Input: part model. Units: mm. Frame: model coordinates. Coordinates: 2 decimals unless noted, no trailing zeros. Write each loop counter-clockwise with the first axis right and the second up, starting at its lowest first coordinate (ties: lowest second). Pieces come first, ordered by that corner, then holes. Notation, with made-up numbers: (-12, 29.5) - (1, 29.5) arc R26 ccw to (1, 66.5) - close; hole circle Ø3 at (37.5, -26.75). An arc over 180 degrees is marked (long way). Put each result on its own line as item: value. Start each with the question number.
1. Line query: line 1 (Y direction, x = 2.75, z = -0.25); line 2 (X direction, y = 2, z = -8) (3 decimals); line 3 (Z direction, x = 1, y = 28.5). Output: solid intervals per line, ascending.
2. Pin query (flat end, axial travel): pin 1 (1.5 mm diameter, centred on x = 2, z = -4, fed in from -Y) (3 decimals). Return the tip coordinate at first contact, or that it passes through.
3. Cut plane A-A, the plane x = 1.3. Return loops of the section in (y, z).
4. Cut plane B-B, the plane y = 29. Return loops of the section in (x, z) (1 decimal), and give its area (3 significant figures).
5. Cut plane C-C, the plane z = -2.25. Return loops of the section in (x, y) (3 decimals).
6. Cut plane D-D, the plane y = 17. Return loops of the section in (x, z) (3 decimals), and give its area (3 significant figures).
from build123d import *

# Parameters (mm, degrees)
BOSS_EXTRUDE1_DEPTH = 31.75
SKETCH7_W           = 3.6195
SKETCH7_H           = 6.35
CUT_EXTRUDE2_DEPTH  = 3.8575
SKETCH10_W          = 3.6195
SKETCH10_H          = 6.35
CUT_EXTRUDE4_DEPTH  = 3.8575
SKETCH15_R          = 1.6383
CUT_EXTRUDE5_DEPTH  = 3.8575


with BuildPart() as part:
    # Sketch3 → Boss-Extrude1 (new body)
    with BuildSketch(Plane(origin=(0, 0, 0), x_dir=(1, 0, 0), z_dir=(0, 1, 0))):
        with BuildLine():
            Line((0.635, 9.525), (0, 9.525))
            Line((0, 9.525), (0, 0))
            ThreePointArc((0, 0), (2.652258403, -0.737803327), (0.762, 1.263634045))
            Line((0.762, 1.263634045), (0.762, 0.430677954))
            ThreePointArc((0.762, 0.430677954), (2.190088254, -0.224506403), (0.635, 0))
            Line((0.635, 0), (0.635, 9.525))
        make_face()
    extrude(amount=BOSS_EXTRUDE1_DEPTH)

    # Sketch7 → Cut-Extrude2 (cut, through all)
    with BuildSketch(Plane(origin=(0, 0, 0), x_dir=(0, 0, -1), z_dir=(1, 0, 0))):
        with Locations((0, 34.925)):
            Rectangle(SKETCH7_W, SKETCH7_H)
        with Locations((0, 9.525)):
            Rectangle(SKETCH7_W, SKETCH7_H)
        with Locations((0, 22.225)):
            Rectangle(SKETCH7_W, SKETCH7_H)
    extrude(amount=CUT_EXTRUDE2_DEPTH, mode=Mode.SUBTRACT)

    # Sketch10 → Cut-Extrude4 (cut, through all)
    with BuildSketch(Plane(origin=(0, 0, 0), x_dir=(0, 0, -1), z_dir=(1, 0, 0))):
        with Locations((0, 15.875)):
            Rectangle(SKETCH10_W, SKETCH10_H)
    extrude(amount=CUT_EXTRUDE4_DEPTH, mode=Mode.SUBTRACT)

    # Sketch15 → Cut-Extrude5 (cut, through all)
    with BuildSketch(Plane(origin=(0, 0, 0), x_dir=(0, 0, -1), z_dir=(1, 0, 0))):
        with Locations((5.9436, 3.175)):
            Circle(SKETCH15_R)
    cut_extrude5 = extrude(amount=CUT_EXTRUDE5_DEPTH, mode=Mode.SUBTRACT)

    # Mirror1: Cut-Extrude5 across plane
    add(cut_extrude5.mirror(Plane(origin=(0, 15.875, 0), x_dir=(0, 0, 1), z_dir=(0, -1, 0))), mode=Mode.SUBTRACT)


solid = part.part
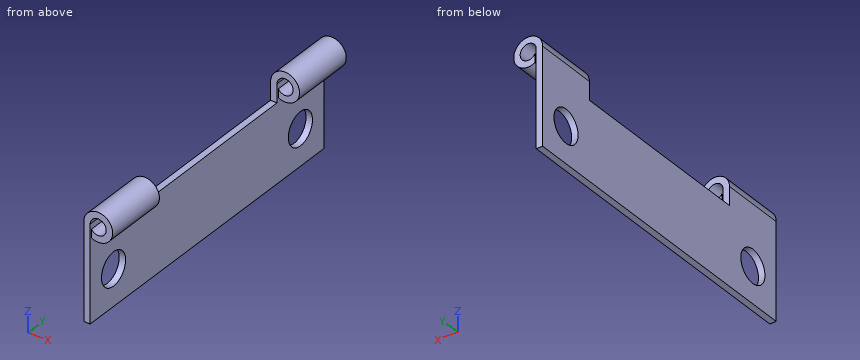
Report:
1. line 1: y = 0 to 6.35, 25.4 to 31.75
1. line 2: x = 0 to 0.635
1. line 3: z = -1.36 to -0.67, 0.67 to 1.36
2. pin 1: passes through
3. outline: (0, -1.42) - (6.35, -1.42) - (6.35, -0.78) - (0, -0.78) - close; (0, 0.78) - (6.35, 0.78) - (6.35, 1.42) - (0, 1.42) - close; (25.4, -1.42) - (31.75, -1.42) - (31.75, -0.78) - (25.4, -0.78) - close; (25.4, 0.78) - (31.75, 0.78) - (31.75, 1.42) - (25.4, 1.42) - close
4. outline: (0, -9.5) - (0.6, -9.5) - (0.6, -7.5) - (0, -7.5) - close; (0, -4.4) - (0.6, -4.4) - (0.6, 0) arc R0.8 cw (long way) to (0.8, -0.4) - (0.8, -1.3) arc R1.4 ccw (long way) to (0, 0) - close
4. area: 7.82 mm^2
5. outline: (0, 0) - (0.635, 0) - (0.635, 31.75) - (0, 31.75) - close
6. outline: (0, -9.525) - (0.635, -9.525) - (0.635, -1.81) - (0, -1.81) - close
6. area: 4.90 mm^2
